Geometry: see drawing. Coordinates: mm, zero at the bounding-box minimum. A direction names the side the tool comes from. Round coordinates to 2 decimals unless told otherwise and drop trailing zeros. Order: outer loops, then holes, each group sorted by start corner. A loop starts at its lowest first (then second) coordinate and runs counter-clockwise, first axis right, second up.
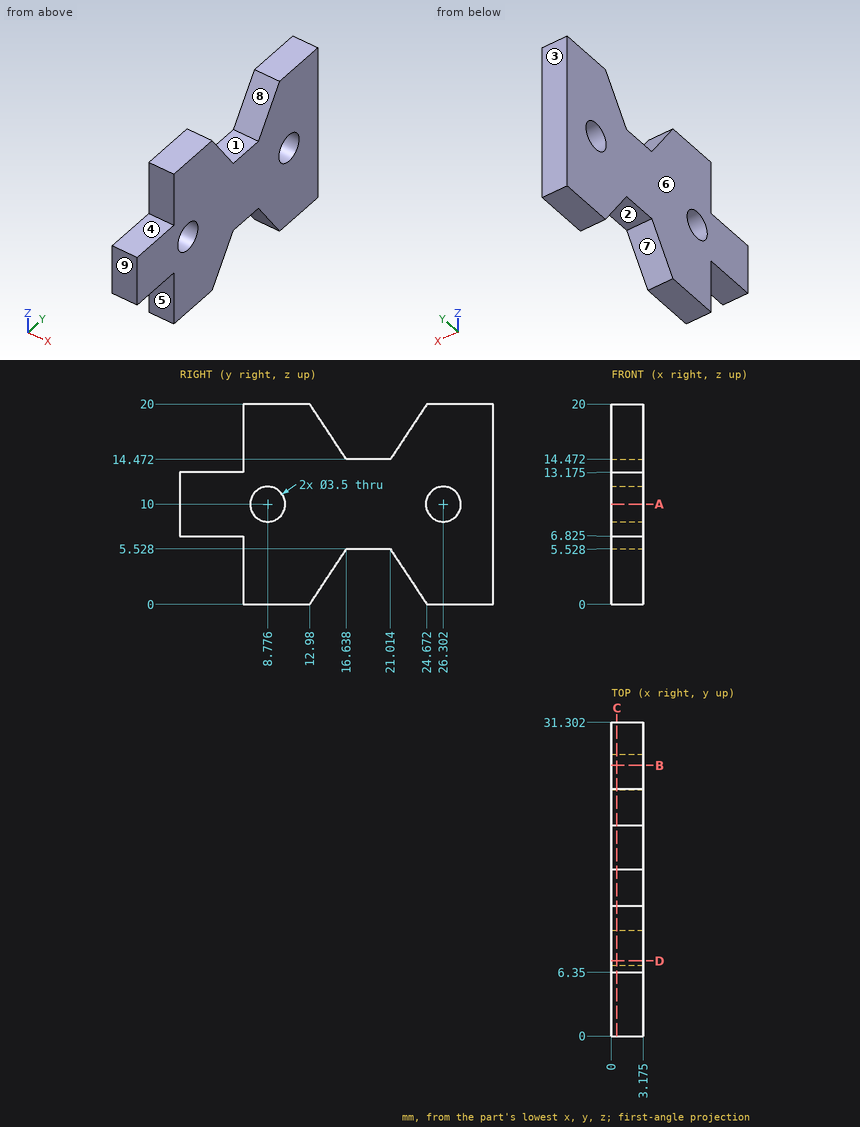
1. Section C-C on x = 0.55. State how many separate pieces and enclosed holes the cut face has, plus the area to 3 significant figures.
2. Section D-D on y = 7.5. Return loops of the section in (x, z) (1 decimal).
3. Access query for the marked faces 1, 2, 3, 4 and 5. Directions: +Z, -Z, +X, -X, +Y, -Y. A direction counts if a zero-diameter tool reaches every point of the face in a straight line with its end or side. Return the directions, or none.
4. Line query: line 1 along Y through (x, z) = (2, 10) (1 decimal); line 2 along Z through (x, y) = (2.2, 27.5) (1 decimal); line 3 along Y through (x, z) = (0.85, 13.5). Output: solid intervals per line, ascending.
5. Pull-direction query (Y, two-part tool) for the marked faces 6, 7, 8 and 9; classes: released by +Y, released by -Y, zero draft, split by the parting line, or undercut.
6. First-contact query: pin 1 (1.6 mm diameter, centred on x = 2, y = 19.5, fed in from -Z); pin 2 (1.6 mm diameter, centred on x = 2.5, y = 19.5, fed in from +Z). Flat tips, straight axial feed; report the tip coordinate or a pass-through.
7. Section B-B on y = 27. Return loops of the section in (x, z) (1 decimal).
8. Section A-A on z = 10. Return loops of the section in (x, y) (1 decimal).
Result:
1. separate pieces: 1
1. enclosed holes: 2
1. area: 431 mm2
2. outline: (0, 0) - (3.2, 0) - (3.2, 8.8) - (0, 8.8) - close; (0, 11.2) - (3.2, 11.2) - (3.2, 20) - (0, 20) - close
3. face 1: +Z, +X, -X
3. face 2: -Z, +X, -X
3. face 3: +Z, -Z, +X, -X, +Y
3. face 4: +Z, +X, -X, -Y
3. face 5: -Z, +X, -X, -Y
4. line 1: y = 0 to 7, 10.5 to 24.6, 28.1 to 31.3
4. line 2: z = 0 to 8.7, 11.3 to 20
4. line 3: y = 6.35 to 31.3
5. face 6: zero draft
5. face 7: undercut
5. face 8: undercut
5. face 9: released by -Y
6. pin 1: stops at z = 5.53
6. pin 2: stops at z = 14.47
7. outline: (0, 0) - (3.2, 0) - (3.2, 8.4) - (0, 8.4) - close; (0, 11.6) - (3.2, 11.6) - (3.2, 20) - (0, 20) - close
8. outline: (0, 0) - (3.2, 0) - (3.2, 7) - (0, 7) - close; (0, 10.5) - (3.2, 10.5) - (3.2, 24.6) - (0, 24.6) - close; (0, 28.1) - (3.2, 28.1) - (3.2, 31.3) - (0, 31.3) - close
